```python
from build123d import *

# Parameters (mm, degrees)
BOSS_EXTRUDE1_DEPTH               = 57.15
SKETCH15_W                        = 50.8
SKETCH15_H                        = 384.175
BOSS_EXTRUDE7_DEPTH               = 36.5125
M8_CLEARANCE_HOLE1_D              = 8.4328
M8_CLEARANCE_HOLE1_DEPTH          = 24.3586
M8_CLEARANCE_HOLE1_TIP            = 2.533468714
FILLET1_R                         = 5.08
F_3_4_NPT_TAPPED_HOLE1_AT_2_COUNT = 2
F_3_4_NPT_TAPPED_HOLE1_AT_2_PITCH = 311.15


with BuildPart() as part:
    # Sketch1 → Boss-Extrude1 (new body)
    with BuildSketch(Plane(origin=(-28.575, 0, 0), x_dir=(0, -1, 0), z_dir=(-1, 0, 0))):
        Polygon((195.2625, 13.49375), (-195.2625, 26.9875), (-195.2625, 0), (195.2625, 0), align=None)
    extrude(amount=-BOSS_EXTRUDE1_DEPTH)

    # Sketch15 → Boss-Extrude7 (add)
    with BuildSketch(Plane(origin=(0, 0, 0), x_dir=(-1, 0, 0), z_dir=(0, 0, -1))):
        Rectangle(SKETCH15_W, SKETCH15_H)
    extrude(amount=BOSS_EXTRUDE7_DEPTH)

    # M8 Clearance Hole1
    with Locations(Plane(origin=(0, 0, -36.5125), x_dir=(-1, 0, 0), z_dir=(0, 0, -1))):
        with Locations((0, 100.0125), (0, -122.2375)):
            Hole(M8_CLEARANCE_HOLE1_D / 2, depth=M8_CLEARANCE_HOLE1_DEPTH)
            with Locations((0, 0, -(M8_CLEARANCE_HOLE1_DEPTH + M8_CLEARANCE_HOLE1_TIP / 2))):  # 118° drill point
                Cone(0, M8_CLEARANCE_HOLE1_D / 2, M8_CLEARANCE_HOLE1_TIP, mode=Mode.SUBTRACT)

    # Fillet1
    fillet1_edges = [part.edges().sort_by_distance(p)[0] for p in [
        (28.575, 195.2625, 13.49375),
        (28.575, -195.2625, 6.746875),
        (-28.575, 195.2625, 13.49375),
        (-28.575, -195.2625, 6.746875),
    ]]
    fillet(fillet1_edges, radius=FILLET1_R)

    # Sketch27 → 3/4 NPT Tapped Hole1 (revolve, cut)
    with BuildSketch(Plane(origin=(0, 144.4625, -36.5125), x_dir=(0, 1, 0), z_dir=(1, 0, 0))):
        Polygon((0, 0), (0, 30.027622455), (11.5062, 23.114), (11.5062, 14.0462), (12.914209362, 14.0462), (13.3347714, 0), align=None)
    f_3_4_npt_tapped_hole1 = revolve(axis=Axis((0, 144.4625, -42.8625), (0, 0, 1)), mode=Mode.SUBTRACT)

    # 3/4 NPT Tapped Hole1 at 2: 3/4 NPT Tapped Hole1 ×2
    with Locations(*[(0, -i * F_3_4_NPT_TAPPED_HOLE1_AT_2_PITCH, 0) for i in range(1, F_3_4_NPT_TAPPED_HOLE1_AT_2_COUNT)]):
        add(f_3_4_npt_tapped_hole1, mode=Mode.SUBTRACT)


solid = part.part
```
Source: CAD feature listing. Evaluate the final solid. Frame: model axes, mm. A direction names the side the tool comes from. Coordinates: 2 decimals unless noted, no trailing zeros. Loops run counter-clockwise (first coordinate to the right, second up) from the corner with the lowest first, then second, coordinate; pieces in that order, holes last. Notation, with made-up numbers: M -10.75,53.5 L -4.75,53.5 A26 cw -4.75,88.5 Z; hole C -7,71 d3. An arc over 180 degrees is marked long. Use a Markdown table: item, result. Add a question column.
Q1. Section query A-A, the plane z = -28. Return loops of the section in (x, y).
Q2. Draft query along X for faces 1 (the flat face through (28.575, 3, 11)), 2 (the flat face through (0, -192.088, -18)), 3 (the conical face through (-3.943, -154.166, -29.588)). Return one class per face: pulls with the +X half, pulls with the -X half, needs draft (parallel to the pull), parting line crosses it, or undercut.
Q3. Section query C-C, the plane y = -84. Return loops of the section in (x, z) (1 decimal).
Q4. Material intervals for L1, parallel to Y at x = 0, z = -17; L2, parallel to Y at x = 0, z = -30.5; L3, parallel to X at y = -121.5, z = -28, sorted ascending.
Q5. Section query B-B, the plane x = 17. Return loops of the section in (y, z).
Q6. First-contact query: pin 1 (11 mm diameter, centred on y = -77.5, z = -27, fed in from -X); pin 2 (4 mm diameter, centred on x = -19.5, z = -20, fed in from -Y); pin 3 (6.5 mm diameter, centred on x = 0, y = -122.24, fed in from +Z). Flat tips, straight axial feed; report the tip coordinate or a pass-through.
Q7. Access query for faces 4 (the flat face through (0, 192.088, -18)), 5 (the flat face through (-25.4, -3, -18)), 6 (the cylindrical face through (-0.914, -126.354, -24.163)). Directions: +Z, -Z, +X, -X, +Y, -Y. A direction counts if a zero-diameter tool reaches every point of the face in a straight line with its end or side. Return the directions, or none.
Q8. Section query D-D, the plane z = 18.5. Return loops of the section in (x, y) (1 decimal).
Result:
| question | item | result |
|---|---|---|
| 1 | outline | M -25.4,-192.09 L 25.4,-192.09 L 25.4,192.09 L -25.4,192.09 Z; hole C 0,-166.69 d26.16; hole C 0,144.46 d26.16; hole C 0,-122.24 d8.43; hole C 0,100.01 d8.43 |
| 2 | face 1 | pulls with the +X half |
| 2 | face 2 | needs draft |
| 2 | face 3 | undercut |
| 3 | outline | M -28.6,0 L -25.4,0 L -25.4,-36.5 L 25.4,-36.5 L 25.4,0 L 28.6,0 L 28.6,17.3 L -28.6,17.3 Z |
| 4 | L1 | y = -192.09 to -178.19, -155.18 to -126.45, -118.02 to 95.8, 104.23 to 132.96, 155.97 to 192.09 |
| 4 | L2 | y = -192.09 to -179.84, -153.53 to -126.45, -118.02 to 95.8, 104.23 to 131.31, 157.62 to 192.09 |
| 4 | L3 | x = -25.4 to -4.15, 4.15 to 25.4 |
| 5 | outline | M -195.26,0 L -192.09,0 L -192.09,-36.51 L 192.09,-36.51 L 192.09,0 L 195.26,0 L 195.26,26.99 L -195.26,13.49 Z |
| 6 | pin 1 | stops at x = -25.4 |
| 6 | pin 2 | stops at y = -192.09 |
| 6 | pin 3 | stops at z = 16.13 |
| 7 | face 4 | -Z, +X, -X, +Y |
| 7 | face 5 | -Z, -X, +Y, -Y |
| 7 | face 6 | -Z |
| 8 | outline | M -28.6,-50.4 L 28.6,-50.4 L 28.6,190.2 A5.1 ccw 23.5,195.3 L -23.5,195.3 A5.1 ccw -28.6,190.2 Z |
